from build123d import *

# Parameters (mm, degrees)
SKETCH1_W           = 580
SKETCH1_H           = 30
BOSS_EXTRUDE1_DEPTH = 7.5
SKETCH2_R           = 10
CUT_EXTRUDE1_DEPTH  = 20
SKETCH3_W           = 40
SKETCH3_H           = 40
SKETCH3_R           = 10
BOSS_EXTRUDE2_DEPTH = 15


with BuildPart() as part:
    # Sketch1 → Boss-Extrude1 (new body, symmetric)
    with BuildSketch(Plane.XY):
        Rectangle(SKETCH1_W, SKETCH1_H)
    extrude(amount=BOSS_EXTRUDE1_DEPTH, both=True)

    # Sketch2 → Cut-Extrude1 (cut)
    with BuildSketch(Plane.XY.offset(7.5)):
        Circle(SKETCH2_R)
    extrude(amount=-CUT_EXTRUDE1_DEPTH, mode=Mode.SUBTRACT)

    # Sketch3 → Boss-Extrude2 (add)
    with BuildSketch(Plane.XY.offset(7.5)):
        with Locations((-170, -35)):
            Rectangle(SKETCH3_W, SKETCH3_H)
        with Locations((-170, -35)):
            Circle(SKETCH3_R, mode=Mode.SUBTRACT)
    extrude(amount=-BOSS_EXTRUDE2_DEPTH)


solid = part.part
Part model, mm, in its own coordinate system. A direction names the side the tool comes from. Coordinates: 2 decimals unless noted, no trailing zeros. Write each loop counter-clockwise with the first axis right and the second up, starting at its lowest first coordinate (ties: lowest second). Pieces come first, ordered by that corner, then holes. Notation, with made-up numbers: (51, 14.5) - (56, 14.5) arc R36 cw to (56, 52.5) - close; hole circle Ø2 at (33, 11). An arc over 180 degrees is marked (long way). Put each result on its own line as item: value.
1. Probe line 1 along Y through (x, z) = (-170, 0.5); line 2 along X through (y, z) = (0.5, -3.25); line 3 along X through (y, z) = (-6.5, 1.5). List the from-to ranges inside material, lowest first. Write a range as [from, to].
Final values:
line 1: y = [-55, -45], [-25, 15]
line 2: x = [-290, -9.99], [9.99, 290]
line 3: x = [-290, -7.6], [7.6, 290]
2. 3-axis set-ups, long thin cutter, end or side, ignore diameter. For faces 5 (the flat face through (-4, -12, -7.5)), 6 (the flat face through (-150, -35, 0)), 7 (the flat face through (-190, -35, 0)): which of +Z, -Z, +X, -X, +Y, -Y reach the whole face in a straight line?
Final values:
face 5: -Z, +X, -X, +Y, -Y
face 6: +Z, -Z, +X, -Y
face 7: +Z, -Z, -X, -Y
3. Band-saw the part on B-B (z = 4.25). Write the cut outline in (x, y).
Final values:
outline: (-290, -15) - (-190, -15) - (-190, -55) - (-150, -55) - (-150, -15) - (290, -15) - (290, 15) - (-290, 15) - close; hole circle Ø20 at (-170, -35); hole circle Ø20 at (0, 0)
4. Band-saw the part on C-C (x = 0). Write the cut outline in (y, z), then the cut area to 3 significant figures.
Final values:
outline: (-15, -7.5) - (-10, -7.5) - (-10, 7.5) - (-15, 7.5) - close; (10, -7.5) - (15, -7.5) - (15, 7.5) - (10, 7.5) - close
area: 150 mm²
5. Band-saw the part on D-D (x = 234.5). Write the cut outline in (y, z).
Final values:
outline: (-15, -7.5) - (15, -7.5) - (15, 7.5) - (-15, 7.5) - close
6. Band-saw the part on A-A (y = -35). Write the cut outline in (x, z).
Final values:
outline: (-190, -7.5) - (-180, -7.5) - (-180, 7.5) - (-190, 7.5) - close; (-160, -7.5) - (-150, -7.5) - (-150, 7.5) - (-160, 7.5) - close
7. Two-plate mould, pull along Y, no slides. Class faces 1 (the cylindrical face through (-2.17, -9.76, 0.11)), 2 (the flat face through (-4, -12, 7.5)), 3 (the flat face through (-4, 15, 0)), 4 (the flat face through (-241, -15, 0)): +Y half, -Y half, draft (parallel to the pull), parting line (faces both ways), or undercut.
Final values:
face 1: undercut
face 2: draft
face 3: +Y half
face 4: -Y half
8. Flat gauge pins, fed straight in: pin 1 Ø12 at (x, y) = (0, 0) entering from -Z; pin 2 Ø3 at (y, z) = (-30, -0.5) entering from +X; pin 3 Ø4 at (y, z) = (-35, 5.5) entering from -X; pin 4 Ø1 at (x, z) = (120.5, 0.5) entering from -Y. Where does each tip first touch, or does it go through?
Final values:
pin 1: passes through
pin 2: stops at x = -150
pin 3: stops at x = -190
pin 4: stops at y = -15
